from build123d import *
from build123d.topology import SkipClean

# Parameters (mm, degrees)
SKETCH1_R                     = 45
BOSS_EXTRUDE1_DEPTH           = 118
SKETCH2_R                     = 17.5
SKETCH2_R_2                   = 7.5
BOSS_EXTRUDE2_DEPTH           = 50
SKETCH3_W                     = 90
SKETCH3_H                     = 118
BOSS_EXTRUDE3_DEPTH           = 10
SKETCH3_2_W                   = 90
SKETCH3_2_H                   = 118
BOSS_EXTRUDE4_DEPTH           = 6
BOSS_EXTRUDE4_TAPER           = 77
BOSS_EXTRUDE4_OTHER_WAY_DEPTH = 6
BOSS_EXTRUDE4_OTHER_WAY_TAPER = 77


with BuildPart() as part:
    # Sketch1 → Boss-Extrude1 (new body)
    with BuildSketch(Plane.XY):
        Circle(SKETCH1_R)
    extrude(amount=BOSS_EXTRUDE1_DEPTH)

    # Sketch2 → Boss-Extrude2 (add)
    with BuildSketch(Plane.XY.offset(118)):
        Circle(SKETCH2_R)
        Circle(SKETCH2_R_2, mode=Mode.SUBTRACT)
    extrude(amount=BOSS_EXTRUDE2_DEPTH)



with BuildPart() as body_2:
    # Sketch3 → Boss-Extrude3 (new body)
    with BuildSketch(Plane(origin=(0, -45, 0), x_dir=(-1, 0, 0), z_dir=(0, -1, 0))):
        with Locations((0, -59)):
            Rectangle(SKETCH3_W, SKETCH3_H)
    extrude(amount=BOSS_EXTRUDE3_DEPTH)


with BuildPart() as part_1:
    add(part.part)

    add(body_2.part)  # Boss-Extrude4 merges body 2
    # Sketch3<2> → Boss-Extrude4 (add)
    with BuildSketch(Plane(origin=(0, -45, 0), x_dir=(-1, 0, 0), z_dir=(0, -1, 0))):
        with Locations((0, -59)):
            Rectangle(SKETCH3_2_W, SKETCH3_2_H)
    extrude(amount=BOSS_EXTRUDE4_DEPTH, taper=BOSS_EXTRUDE4_TAPER)

    # Sketch3<2> → Boss-Extrude4 other way (add)
    with SkipClean():  # the faces are left unmerged after this step: merging them gives an invalid solid
        with BuildSketch(Plane(origin=(0, -45, 0), x_dir=(-1, 0, 0), z_dir=(0, -1, 0))):
            with Locations((0, -59)):
                Rectangle(SKETCH3_2_W, SKETCH3_2_H)
        extrude(amount=-BOSS_EXTRUDE4_OTHER_WAY_DEPTH, taper=BOSS_EXTRUDE4_OTHER_WAY_TAPER)


solid = part_1.part
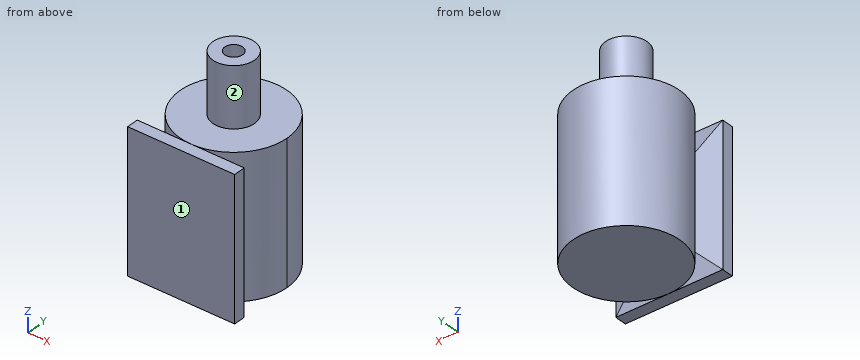
Geometry: final body of the model. Coordinates: model frame, mm. Face numbers are marked on the shaded views. A direction names the side the tool comes from. Coordinates: 2 decimals unless noted, no trailing zeros. Order: outer loops, then holes, each group sorted by start corner. A loop starts at its lowest first (then second) coordinate and runs counter-clockwise, first axis right, second up.
1) Ray query, probe 1 along Y at (x, z) = (0, 143); probe 2 along Z at (x, y) = (15.5, -46.5); probe 3 along Y at (x, z) = (37, 99.5). Return the intervals inside material, ascending.
Result sheet:
probe 1: y = -17.5 to -7.5, 7.5 to 17.5
probe 2: z = 0 to 118
probe 3: y = -55 to -43.15, -25.61 to 25.61
2) Set-up query: the marked faces 1 and 2. Return all of +Z, -Z, +X, -X, +Y, -Y with unobstructed straight access to the full face (end or side cutting, diameter ignored); none if empty.
Result sheet:
face 1: +Z, -Z, +X, -X, -Y
face 2: +Z
3) First-contact query: P1, Ø4, axis at x = -18, z = 147, coming from the -Y side; P2, Ø12, axis at x = 0, y = 0, coming from the +Z side; P3, Ø1, axis at y = -6.5, z = 42.5, coming from the +X side. Flat tips, straight axial feed; report the tip coordinate or a pass-through.
Result sheet:
P1: stops at y = -7.09
P2: stops at z = 118
P3: stops at x = 44.6
4) Section B-B (y = 20). Return loops of the section in (x, z).
Result sheet:
outline: (-40.31, 0) - (40.31, 0) - (40.31, 118) - (-40.31, 118) - close
5) Section C-C (y = -24.5). Return loops of the section in (x, z), then the cut area to 3 significant figures.
Result sheet:
outline: (-37.75, 0) - (37.75, 0) - (37.75, 118) - (-37.75, 118) - close
area: 8,910 mm2
6) Section A-A (y = 4.5). Return loops of the section in (x, z).
Result sheet:
outline: (-44.77, 0) - (44.77, 0) - (44.77, 118) - (16.91, 118) - (16.91, 168) - (6, 168) - (6, 118) - (-6, 118) - (-6, 168) - (-16.91, 168) - (-16.91, 118) - (-44.77, 118) - close
